from build123d import *

# Parameters (mm, degrees)
SKETCH1_W               = 200
SKETCH1_H               = 200
BOSS_EXTRUDE1_DEPTH     = 55
FILLET1_R               = 20
SKETCH2_W               = 210
SKETCH2_H               = 210
SKETCH2_W_2             = 200
SKETCH2_H_2             = 200
BOSS_EXTRUDE2_DEPTH     = 12
SKETCH3_W               = 210
SKETCH3_H               = 210
BOSS_EXTRUDE3_DEPTH     = 12
CUT_EXTRUDE1_DEPTH      = 159.350876221
CUT_EXTRUDE1_DEPTH_BACK = 159.350876221
SKETCH5_W               = 180
SKETCH5_H               = 180
CHAMFER1_SIZE           = 2
FILLET2_R               = 10
FILLET3_R               = 3
FILLET4_R               = 20


with BuildPart() as part:
    # Sketch1 → Boss-Extrude1 (new body)
    with BuildSketch(Plane(origin=(0, 0, 0), x_dir=(1, 0, 0), z_dir=(0, 1, 0))):
        Rectangle(SKETCH1_W, SKETCH1_H)
    extrude(amount=-BOSS_EXTRUDE1_DEPTH)

    # Fillet1
    fillet1_edges = [part.edges().sort_by_distance(p)[0] for p in [
        (100, -27.5, 100),
        (-100, -27.5, 100),
        (-100, -27.5, -100),
        (100, -27.5, -100),
    ]]
    fillet(fillet1_edges, radius=FILLET1_R)

    # Sketch3 → Boss-Extrude3 (add)
    with BuildSketch(Plane(origin=(0, 0, 0), x_dir=(1, 0, 0), z_dir=(0, 1, 0))):
        Rectangle(SKETCH3_W, SKETCH3_H)
    extrude(amount=-BOSS_EXTRUDE3_DEPTH)


with BuildPart() as body_2:
    # Sketch2 → Boss-Extrude2 (new body)
    with BuildSketch(Plane(origin=(0, 0, 0), x_dir=(1, 0, 0), z_dir=(0, 1, 0))):
        Rectangle(SKETCH2_W, SKETCH2_H)
        Rectangle(SKETCH2_W_2, SKETCH2_H_2, mode=Mode.SUBTRACT)
    extrude(amount=BOSS_EXTRUDE2_DEPTH)

    # Combine2: union part
    add(part.part)

    # Sketch5 → Cut-Extrude1 (cut, two sides: drawn at the far end of the back side and taken through both)
    with BuildSketch(Plane(origin=(0, 0, 0), x_dir=(1, 0, 0), z_dir=(0, 1, 0)).offset(-CUT_EXTRUDE1_DEPTH_BACK)):
        Rectangle(SKETCH5_W, SKETCH5_H)
    extrude(amount=CUT_EXTRUDE1_DEPTH + CUT_EXTRUDE1_DEPTH_BACK, mode=Mode.SUBTRACT)

    # Chamfer1
    chamfer1_edges = [body_2.edges().sort_by_distance(p)[0] for p in [
        (-105, 12, 0),
        (100, 12, 0),
        (0, 12, 105),
        (0, 12, -100),
        (-100, 12, 0),
        (0, 12, 100),
        (105, 12, 0),
        (0, 12, -105),
    ]]
    chamfer(chamfer1_edges, length=CHAMFER1_SIZE)

    # Fillet2
    # the kernel refuses this fillet: 10 mm, written as the material it takes off along each edge
    with BuildSketch(Plane(origin=(105, 35, 105), x_dir=(-1, 0, 0), z_dir=(0, -1, 0)), Plane(origin=(-105, 35, 105), x_dir=(0, 0, -1), z_dir=(0, -1, 0)), Plane(origin=(-105, -37, -105), x_dir=(0, 0, 1), z_dir=(0, 1, 0))) as fillet2_piece_1:
        with BuildLine():
            CenterArc((FILLET2_R, FILLET2_R), FILLET2_R, 180, 90)
            Line((0, FILLET2_R), (0, 0))
            Line((0, 0), (FILLET2_R, 0))
        make_face()
    extrude(amount=72, mode=Mode.SUBTRACT)
    with BuildSketch(Plane(origin=(105, 35, -105), x_dir=(-1, 0, 0), z_dir=(0, -1, 0))) as fillet2_piece_2:
        with BuildLine():
            CenterArc((FILLET2_R, -FILLET2_R), FILLET2_R, 90, 90)
            Line((0, -FILLET2_R), (0, 0))
            Line((0, 0), (FILLET2_R, 0))
        make_face()
    extrude(amount=72, mode=Mode.SUBTRACT)

    # Fillet3
    fillet3_edges = [body_2.edges().sort_by_distance(p)[0] for p in [
        (100, -55, 0),
        (0, -55, 100),
        (-100, -55, 0),
        (0, -55, -100),
        (94.142135624, -55, -94.142135624),
        (94.142135624, -55, 94.142135624),
        (-94.142135624, -55, 94.142135624),
        (-94.142135624, -55, -94.142135624),
        (0, -12, -100),
        (-94.142135624, -12, -94.142135624),
        (-100, -12, 0),
        (-94.142135624, -12, 94.142135624),
        (0, -12, 100),
        (94.142135624, -12, 94.142135624),
        (100, -12, 0),
        (94.142135624, -12, -94.142135624),
    ]]
    fillet(fillet3_edges, radius=FILLET3_R)

    # Fillet4
    fillet4_edges = [body_2.edges().sort_by_distance(p)[0] for p in [
        (90, -27.5, -90),
        (90, -27.5, 90),
        (-90, -27.5, 90),
        (-90, -27.5, -90),
    ]]
    fillet(fillet4_edges, radius=FILLET4_R)


solid = body_2.part
Can you work these out from the model? Positions are in its coordinate system, mm. A direction names the side the tool comes from. Give positions to 0.01 mm unless a question says otherwise; leave off trailing zeros. Write each loop counter-clockwise with the first axis right and the second up, starting at its lowest first coordinate (ties: lowest second). Pieces come first, ordered by that corner, then holes. Notation, with made-up numbers: M 0.5,23 L 30.5,23 A25 ccw 30.5,56 Z; hole C -38,60.5 d4. An arc over 180 degrees is marked long. Answer in a Markdown table with one row per item. Add a question column.
Item 1: Imagine slicing it at C-C, the plane z = 22. Write out the boundary of the cut face in (x, y), plus the area to 3 significant figures.
Item 2: On a 3-axis mill with a long thin cutter (end or side, diameter ignored), from which of +Z, -Z, +X, -X, +Y, -Y can I reach the whole of each face in a straight line? I mean faces 4 (the cylindrical face through (-94.297, -33.759, 93.986)), 5 (the flat face through (-1, 5, 100)), 6 (the flat face through (-100, -33, 1)), 7 (the flat face through (-1, -28, 90)). Say none if no direction works.
Item 3: We'd pull the mould along Z, two halves only. Please class faces 1 (the cylindrical face through (-101.99, 0.17, 102.15)), 2 (the flat face through (-1, -33, -100)), 3 (the flat face through (-1, 5, -100)): released by +Z, released by -Z, zero draft, split by the parting line, or undercut.
Item 4: Imagine slicing it at A-A, the plane y = -35. Write out the boundary of the cut face in (x, z), plus the area to 3 significant figures.
Item 5: Imagine slicing it at B-B, the plane x = 4. Write out the boundary of the cut face in (y, z), plus the area to 3 significant figures.
Item 6: Please list where these lines run through material, in increasing order: L1, parallel to X at y = -33, z = 25.5; L2, parallel to X at y = -1.5, z = 67.
Item 7: For pin 1 Ø3 at (x, y) = (27, -46.5) entering from +Z; pin 2 Ø11 at (x, y) = (-30.5, -33) entering from -Z; pin 3 Ø16.5 at (y, z) = (-35, 25.5) entering from +X, each with a flat end and sliding along its axis, tell me the tip position at first contact or that it passes through.
Evaluation:
| question | item | result |
|---|---|---|
| 1 | outline | M -105,-12 L -103,-12 A3 cw -100,-15 L -100,-52 A3 ccw -97,-55 L -90,-55 L -90,0 L -100,0 L -100,10 L -102,12 L -103,12 L -105,10 Z; M 90,-55 L 97,-55 A3 ccw 100,-52 L 100,-15 A3 cw 103,-12 L 105,-12 L 105,10 L 103,12 L 102,12 L 100,10 L 100,0 L 90,0 Z |
| 1 | area | 1,330 mm² |
| 2 | face 4 | +Z, -X, -Y |
| 2 | face 5 | +Y |
| 2 | face 6 | +Z, -Z, -X, -Y |
| 2 | face 7 | +Y, -Y |
| 3 | face 1 | released by +Z |
| 3 | face 2 | released by -Z |
| 3 | face 3 | undercut |
| 4 | outline | M -100,-80 A20 ccw -80,-100 L 80,-100 A20 ccw 100,-80 L 100,80 A20 ccw 80,100 L -80,100 A20 ccw -100,80 Z; hole M -90,-70 A20 ccw -70,-90 L 70,-90 A20 ccw 90,-70 L 90,70 A20 ccw 70,90 L -70,90 A20 ccw -90,70 Z |
| 4 | area | 7,600 mm² |
| 5 | outline | M -55,-97 A3 ccw -52,-100 L -15,-100 A3 cw -12,-103 L -12,-105 L 10,-105 L 12,-103 L 12,-102 L 10,-100 L 0,-100 L 0,-90 L -55,-90 Z; M -55,90 L 0,90 L 0,100 L 10,100 L 12,102 L 12,103 L 10,105 L -12,105 L -12,103 A3 cw -15,100 L -52,100 A3 ccw -55,97 Z |
| 5 | area | 1,330 mm² |
| 6 | L1 | x = -100 to -90, 90 to 100 |
| 6 | L2 | x = -105 to -90, 90 to 105 |
| 7 | pin 1 | stops at z = 100 |
| 7 | pin 2 | stops at z = -100 |
| 7 | pin 3 | stops at x = 100 |
